```python
from build123d import *

# Parameters (mm, degrees)
F2_R     = 1.2
F3_R     = 1.5
F4_DEPTH = 4.001
F5_R     = 1.5
F6_DEPTH = 4.001


with BuildPart() as f1:
    # F0 (on Front) → F1 (revolve)
    with BuildSketch(Plane.XZ):
        Polygon((4.282442, 3.15), (-7.717558, 3.15), (-10.853604, 0.954117), (-10.853604, 0), (7.282442, 0), (7.282442, 4), (4.282442, 4), align=None)
    revolve(axis=Axis((2.625406, 0, 0), (1, 0, 0)))

    # F2
    f2_edges = [f1.edges().sort_by_distance(p)[0] for p in [
        (-10.853604, 0, -0.954117),
        (-7.717558, 0, -3.15),
    ]]
    fillet(f2_edges, radius=F2_R)

    # F3 (on Front) → F4 (cut, through all)
    with BuildSketch(Plane.XZ):
        with Locations((-5.5, 0)):
            Circle(F3_R)
    extrude(amount=F4_DEPTH, mode=Mode.SUBTRACT)

    # F5 (on Front) → F6 (cut, through all)
    with BuildSketch(Plane.XZ):
        with Locations((-5.5, 0)):
            Circle(F5_R)
    extrude(amount=-F6_DEPTH, mode=Mode.SUBTRACT)


solid = f1.part
```
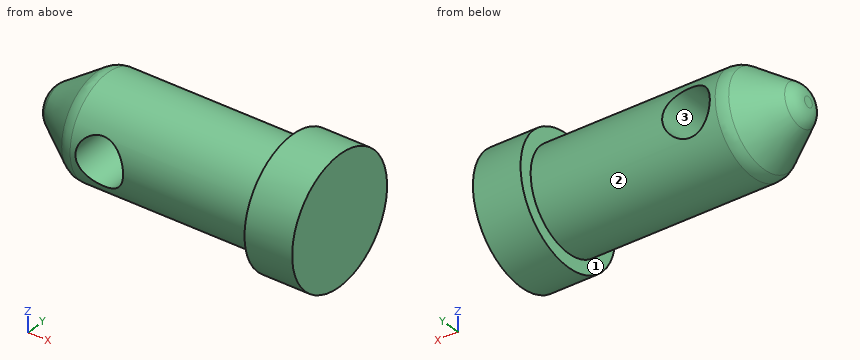
Geometry: final body of the model. Coordinates: model frame, mm. Face numbers are marked on the shaded views. Coordinates: 2 decimals unless noted, no trailing zeros. Order: outer loops, then holes, each group sorted by start corner. A loop starts at its lowest first (then second) coordinate and runs counter-clockwise, first axis right, second up. Notation, with made-up numbers: (75.25, 11.5) - (83.25, 11.5) arc R19 cw to (83.25, 40.5) - close; hole circle Ø10 at (73.25, -13). An arc over 180 degrees is marked (long way). Return JSON: item names as keys, results as strings. Group by question number.
1. Material intervals for line 1 along X through (y, z) = (0.25, 0); line 2 along X through (y, z) = (2, 3); line 3 along X through (y, z) = (1, 0), sorted ascending. Write a range as [from, to].
2. Cut plane B-B (x = 0.75). Output: boundary loops of the cut face in (y, z).
3. Cut plane A-A (x = -5.5). Output: boundary loops of the cut face in (y, z).
4. Pull-direction query (Z, two-part tool) for the marked faces 1, 2 and 3; classes: pulls with the +Z half, pulls with the -Z half, needs draft (parallel to the pull), parting line crosses it, or undercut.
5. Pin query (flat end, axial travel): pin 1 (1 mm diameter, centred on x = -8, y = 2.5, fed in from +Z); pin 2 (2 mm diameter, centred on x = -3, z = -0.5, fed in from -Y); pin 3 (1 mm diameter, centred on y = 1.5, z = 2, fed in from -X). Return the tip coordinate at first contact, or that it passes through.
Resolved:
{
 "1": {"line 1": "x = [-10.85, -7], [-4, 7.28]", "line 2": "x = [4.28, 7.28]", "line 3": "x = [-10.65, -7], [-4, 7.28]"},
 "2": {"outline": "circle Ø6.3 at (0, 0)"},
 "3": {"outline": "(-2.77, -1.5) arc R3.15 ccw to (2.77, -1.5) - close; (-2.77, 1.5) - (2.77, 1.5) arc R3.15 ccw to start"},
 "4": {"face 1": "needs draft", "face 2": "parting line crosses it", "face 3": "undercut"},
 "5": {"pin 1": "stops at z = 2.28", "pin 2": "stops at y = -3.15", "pin 3": "stops at x = -9.36"}
}
